CAD build for the part. Positions are in the model's coordinates, mm. Face numbers are marked on the shaded views. A direction names the side the tool comes from. Round coordinates to 2 decimals unless told otherwise and drop trailing zeros. Order: outer loops, then holes, each group sorted by start corner. A loop starts at its lowest first (then second) coordinate and runs counter-clockwise, first axis right, second up. Notation, with made-up numbers: (-17.75, 5) -> (10.25, 5) arc R13 cw to (10.25, 21) -> close; hole circle Ø11 at (67, -5). An arc over 180 degrees is marked (long way). Return JSON: item names as keys, results as strings. Group by question number.
Q1. Cut at B-B (x = -7.5). Write the cut outline in (y, z).
Q2. Cut at A-A (y = 5). Write the cut outline in (x, z), then the cut area to 3 significant figures.
Q3. Probe line 1 along Z through (x, y) = (-9.5, 4); line 2 along Z through (x, y) = (-16.5, 5.25); line 3 along X through (y, z) = (9, -3). List the from-to ranges inside material, lowest first.
Q4. Flat gauge pins, fed straight in: pin 1 (5.5 mm diameter, centred on x = -6, y = 5.5, fed in from +Z); pin 2 (1.5 mm diameter, centred on x = -3, z = 5, fed in from +Y); pin 3 (10.5 mm diameter, centred on x = -10, z = -7.5, fed in from +Y). Where does each tip first touch, or does it go through?
Q5. Cut at D-D (y = 11.75). Write the cut outline in (x, z).
Q6. Which spindle directions (+Z, -Z, +X, -X, +Y, -Y) get a long thin tool onto all of the face, cutting with end or side? Do the marked faces 5 and 6. Say none if no direction does.
Q7. Cut at C-C (z = -13). Write the cut outline in (x, y).
Q8. Mould opens along Z. For the marked faces 1, 2, 3 and 4 say: +Z half, -Z half, draft (parallel to the pull), parting line (faces both ways), or undercut.
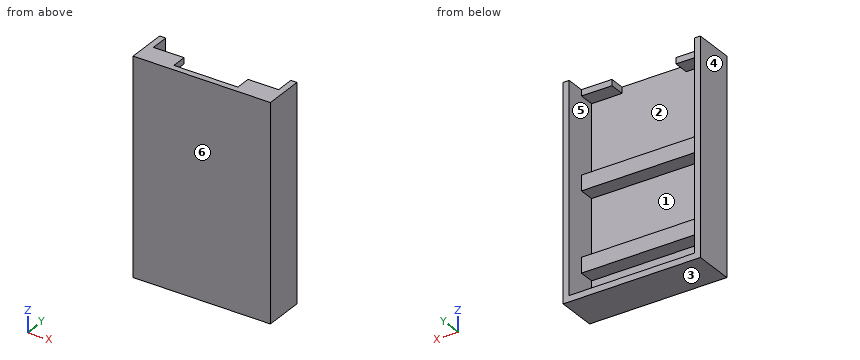
from build123d import *

# Parameters (mm, degrees)
SKETCH1_W               = 45
SKETCH1_H               = 70
BOSS_EXTRUDE1_DEPTH     = 10
SKETCH2_W               = 41
SKETCH2_H               = 66
CUT_EXTRUDE1_DEPTH      = 8
SKETCH7_W               = 41
SKETCH7_H               = 3
CUT_EXTRUDE2_DEPTH      = 1
CUT_EXTRUDE2_DEPTH_BACK = 81
SKETCH8_W               = 21
SKETCH8_H               = 5
CUT_EXTRUDE3_DEPTH      = 42
SKETCH9_W               = 41
SKETCH9_H               = 5
BOSS_EXTRUDE3_DEPTH     = 5
SKETCH10_W              = 41
SKETCH10_H              = 5
BOSS_EXTRUDE4_DEPTH     = 5
SKETCH13_W              = 2
SKETCH13_H              = 70
BOSS_EXTRUDE5_DEPTH     = 3
SKETCH14_W              = 41
SKETCH14_H              = 2
BOSS_EXTRUDE6_DEPTH     = 3
SKETCH15_W              = 2
SKETCH15_H              = 70
BOSS_EXTRUDE7_DEPTH     = 3


with BuildPart() as part:
    # Sketch1 → Boss-Extrude1 (new body)
    with BuildSketch(Plane(origin=(0, 0, 0), x_dir=(1, 0, 0), z_dir=(0, 1, 0))):
        Rectangle(SKETCH1_W, SKETCH1_H)
    extrude(amount=BOSS_EXTRUDE1_DEPTH)

    # Sketch2 → Cut-Extrude1 (cut)
    with BuildSketch(Plane(origin=(0, 10, 0), x_dir=(1, 0, 0), z_dir=(0, 1, 0))):
        Rectangle(SKETCH2_W, SKETCH2_H)
    extrude(amount=-CUT_EXTRUDE1_DEPTH, mode=Mode.SUBTRACT)

    # Sketch7 → Cut-Extrude2 (cut, two sides)
    with BuildSketch(Plane(origin=(0, 0, 33), x_dir=(-1, 0, 0), z_dir=(0, 0, -1))) as cut_extrude2_sk:
        with Locations((0, 8.5)):
            Rectangle(SKETCH7_W, SKETCH7_H)
    extrude(amount=CUT_EXTRUDE2_DEPTH, mode=Mode.SUBTRACT)
    extrude(cut_extrude2_sk.sketch, amount=-CUT_EXTRUDE2_DEPTH_BACK, mode=Mode.SUBTRACT)

    # Sketch8 → Cut-Extrude3 (cut)
    with BuildSketch(Plane(origin=(0, 0, 33), x_dir=(-1, 0, 0), z_dir=(0, 0, -1))):
        with Locations((0, 4.5)):
            Rectangle(SKETCH8_W, SKETCH8_H)
    extrude(amount=-CUT_EXTRUDE3_DEPTH, mode=Mode.SUBTRACT)

    # Sketch9 → Boss-Extrude3 (add)
    with BuildSketch(Plane(origin=(0, 2, 0), x_dir=(1, 0, 0), z_dir=(0, 1, 0))):
        with Locations((0, -5.5)):
            Rectangle(SKETCH9_W, SKETCH9_H)
    extrude(amount=BOSS_EXTRUDE3_DEPTH)

    # Sketch10 → Boss-Extrude4 (add)
    with BuildSketch(Plane(origin=(0, 2, 0), x_dir=(1, 0, 0), z_dir=(0, 1, 0))):
        with Locations((0, 20.5)):
            Rectangle(SKETCH10_W, SKETCH10_H)
    extrude(amount=BOSS_EXTRUDE4_DEPTH)

    # Sketch13 → Boss-Extrude5 (add)
    with BuildSketch(Plane(origin=(0, 10, 0), x_dir=(1, 0, 0), z_dir=(0, 1, 0))):
        with Locations((-21.5, 0)):
            Rectangle(SKETCH13_W, SKETCH13_H)
    extrude(amount=BOSS_EXTRUDE5_DEPTH)

    # Sketch14 → Boss-Extrude6 (add)
    with BuildSketch(Plane(origin=(0, 10, 0), x_dir=(1, 0, 0), z_dir=(0, 1, 0))):
        with Locations((0, 34)):
            Rectangle(SKETCH14_W, SKETCH14_H)
    extrude(amount=BOSS_EXTRUDE6_DEPTH)

    # Sketch15 → Boss-Extrude7 (add)
    with BuildSketch(Plane(origin=(0, 10, 0), x_dir=(1, 0, 0), z_dir=(0, 1, 0))):
        with Locations((21.5, 0)):
            Rectangle(SKETCH15_W, SKETCH15_H)
    extrude(amount=BOSS_EXTRUDE7_DEPTH)


solid = part.part
Solution:
{
 "1": {"outline": "(0, -35) -> (13, -35) -> (13, -33) -> (2, -33) -> (2, -23) -> (7, -23) -> (7, -18) -> (2, -18) -> (2, 3) -> (7, 3) -> (7, 8) -> (2, 8) -> (2, 35) -> (0, 35) -> close"},
 "2": {"outline": "(-22.5, -35) -> (22.5, -35) -> (22.5, 35) -> (10.5, 35) -> (10.5, 33) -> (20.5, 33) -> (20.5, 8) -> (-20.5, 8) -> (-20.5, 33) -> (-10.5, 33) -> (-10.5, 35) -> (-22.5, 35) -> close; hole (-20.5, -33) -> (20.5, -33) -> (20.5, -23) -> (-20.5, -23) -> close; hole (-20.5, -18) -> (20.5, -18) -> (20.5, 3) -> (-20.5, 3) -> close", "area": "812 mm²"},
 "3": {"line 1": "z = -35 to -33, -23 to -18, 3 to 8", "line 2": "z = -35 to -33, -23 to -18, 3 to 8, 33 to 35", "line 3": "x = -22.5 to -20.5, 20.5 to 22.5"},
 "4": {"pin 1": "stops at z = 8", "pin 2": "stops at y = 7", "pin 3": "stops at y = 2"},
 "5": {"outline": "(-22.5, -35) -> (22.5, -35) -> (22.5, 35) -> (20.5, 35) -> (20.5, -33) -> (-20.5, -33) -> (-20.5, 35) -> (-22.5, 35) -> close"},
 "6": {"face 5": "+Y", "face 6": "+Z, -Z, +X, -X, -Y"},
 "7": {"outline": "(-22.5, 0) -> (22.5, 0) -> (22.5, 13) -> (20.5, 13) -> (20.5, 2) -> (-20.5, 2) -> (-20.5, 13) -> (-22.5, 13) -> close"},
 "8": {"face 1": "undercut", "face 2": "undercut", "face 3": "-Z half", "face 4": "draft"}
}
